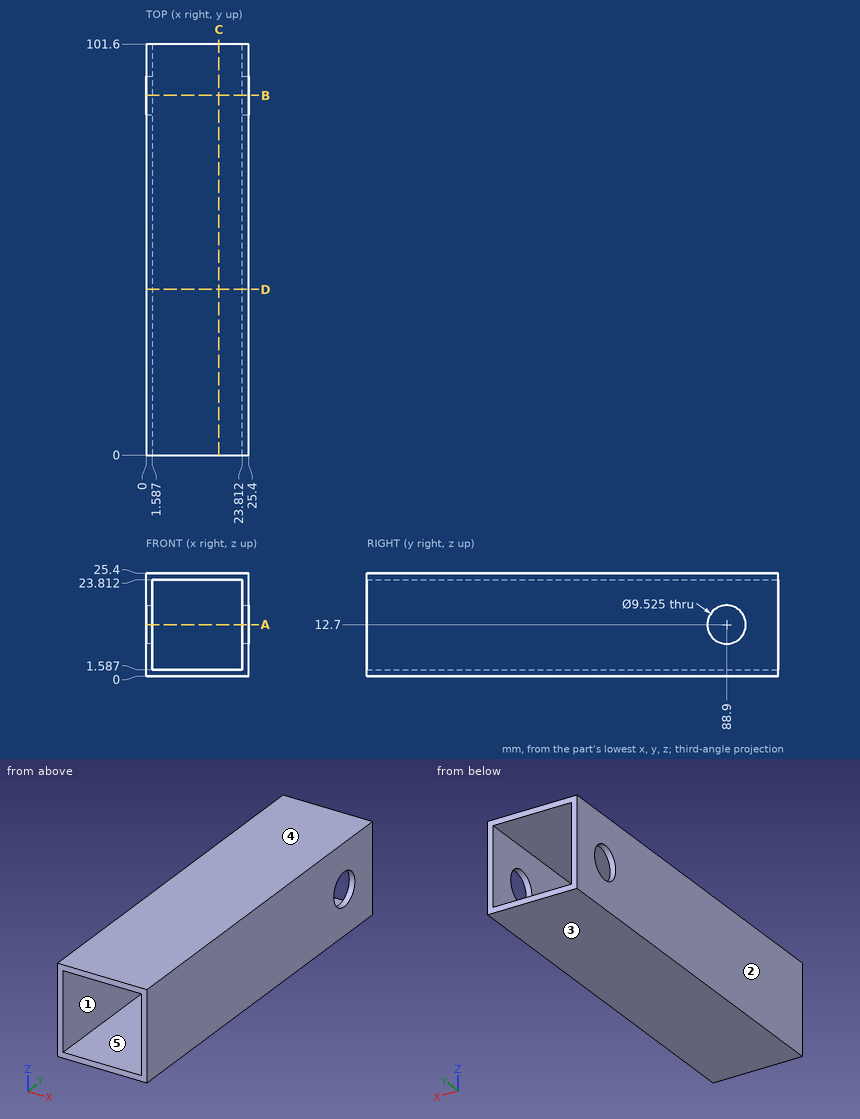
The figure shows three views and two pictorial views of one solid part (mm, origin at its lowest corner). Answer the questions. A direction names the side the tool comes from. Give positions to 0.01 mm unless a question says otherwise; leave off trailing zeros. Order: outer loops, then holes, each group sorted by start corner. A loop starts at its lowest first (then second) coordinate and runs counter-clockwise, first axis right, second up. Notation, with made-up numbers: (60.5, 7.25) - (80.5, 7.25) arc R27 cw to (80.5, 39.25) - close; hole circle Ø10 at (61.25, 57). An arc over 180 degrees is marked (long way). Answer as CSV lines item,"result".
Q1. A cutting plane is placed at A-A, the plane z = 12.7. Determine the outline of the cut face in (x, y).
Answer key:
outline,"(0, 0) - (1.59, 0) - (1.59, 84.14) - (0, 84.14) - close; (0, 93.66) - (1.59, 93.66) - (1.59, 101.6) - (0, 101.6) - close; (23.81, 0) - (25.4, 0) - (25.4, 84.14) - (23.81, 84.14) - close; (23.81, 93.66) - (25.4, 93.66) - (25.4, 101.6) - (23.81, 101.6) - close"
Q2. Determine the mould class of the marked faces 3, 4 and 5 for opening direction Z: pulls with the +Z half, pulls with the -Z half, needs draft (parallel to the pull), parting line crosses it, or undercut.
Answer key:
face 3,"pulls with the -Z half"
face 4,"pulls with the +Z half"
face 5,"undercut"
Q3. Which of the six approach directions +Z, -Z, +X, -X, +Y, -Y give full straight-line access (tool end or side, diameter ignored) to the marked faces 1 and 2?
Answer key:
face 1,"+Y, -Y"
face 2,"+Z, -Z, -X, +Y, -Y"
Q4. A cutting plane is placed at C-C, the plane x = 18. Determine the outline of the cut face in (y, z).
Answer key:
outline,"(0, 0) - (101.6, 0) - (101.6, 1.59) - (0, 1.59) - close; (0, 23.81) - (101.6, 23.81) - (101.6, 25.4) - (0, 25.4) - close"
Q5. A cutting plane is placed at B-B, the plane y = 88.9. Determine the outline of the cut face in (x, z).
Answer key:
outline,"(0, 0) - (25.4, 0) - (25.4, 7.94) - (23.81, 7.94) - (23.81, 1.59) - (1.59, 1.59) - (1.59, 7.94) - (0, 7.94) - close; (0, 17.46) - (1.59, 17.46) - (1.59, 23.81) - (23.81, 23.81) - (23.81, 17.46) - (25.4, 17.46) - (25.4, 25.4) - (0, 25.4) - close"
Q6. This flat-tipped pin is pushed along its axis until it touches: pin 1 Ø8 at (x, z) = (11, 8.5) entering from -Y. Where does it stop, or does it pass through?
Answer key:
pin 1,"passes through"
Q7. Straight lines are drawn through the part: L1, parallel to Z at x = 3, y = 64.5; L2, parallel to Y at x = 24.2, z = 12.7. For each, find the intervals that lie inside material, in ascending order.
Answer key:
L1,"z = 0 to 1.59, 23.81 to 25.4"
L2,"y = 0 to 84.14, 93.66 to 101.6"
Q8. A cutting plane is placed at D-D, the plane y = 41. Determine the outline of the cut face in (x, z), and give its area (3 significant figures).
Answer key:
outline,"(0, 0) - (25.4, 0) - (25.4, 25.4) - (0, 25.4) - close; hole (1.59, 1.59) - (23.81, 1.59) - (23.81, 23.81) - (1.59, 23.81) - close"
area,"151 mm^2"
